from build123d import *

# Parameters (mm, degrees)
SKETCH1_W           = 30
SKETCH1_H           = 36
BOSS_EXTRUDE1_DEPTH = 30
SKETCH3_R           = 12.375
CUT_EXTRUDE1_DEPTH  = 40
SKETCH5_R           = 1.875
CUT_EXTRUDE2_DEPTH  = 40
CUT_EXTRUDE3_START  = 15
SKETCH7_W           = 36
SKETCH7_H           = 15
CUT_EXTRUDE3_DEPTH  = 31
SKETCH8_W           = 9.5
SKETCH8_H           = 22
CUT_EXTRUDE4_DEPTH  = 10


with BuildPart() as part:
    # Sketch1 → Boss-Extrude1 (new body)
    with BuildSketch(Plane(origin=(0, 0, 0), x_dir=(1, 0, 0), z_dir=(0, 1, 0))):
        Rectangle(SKETCH1_W, SKETCH1_H)
    extrude(amount=BOSS_EXTRUDE1_DEPTH)

    # Sketch3 → Cut-Extrude1 (cut)
    with BuildSketch(Plane(origin=(15, 0, 0), x_dir=(0, 0, -1), z_dir=(1, 0, 0))):
        with Locations((0, 15)):
            Circle(SKETCH3_R)
    extrude(amount=-CUT_EXTRUDE1_DEPTH, mode=Mode.SUBTRACT)

    # Sketch5 → Cut-Extrude2 (cut)
    with BuildSketch(Plane(origin=(0, 30, 0), x_dir=(1, 0, 0), z_dir=(0, 1, 0))):
        with Locations((-12.25, 15.25)):
            Circle(SKETCH5_R)
        with Locations((-12.25, -15.25)):
            Circle(SKETCH5_R)
        with Locations((12.25, -15.25)):
            Circle(SKETCH5_R)
        with Locations((12.25, 15.25)):
            Circle(SKETCH5_R)
    extrude(amount=-CUT_EXTRUDE2_DEPTH, mode=Mode.SUBTRACT)

    # Sketch7 → Cut-Extrude3 (cut, through all)
    with BuildSketch(Plane(origin=(0, 0, 0), x_dir=(0, 0, -1), z_dir=(1, 0, 0)).offset(CUT_EXTRUDE3_START)):
        with Locations((0, 7.5)):
            Rectangle(SKETCH7_W, SKETCH7_H)
    extrude(amount=-CUT_EXTRUDE3_DEPTH, mode=Mode.SUBTRACT)

    # Sketch8 → Cut-Extrude4 (cut)
    with BuildSketch(Plane(origin=(0, 30, 0), x_dir=(1, 0, 0), z_dir=(0, 1, 0))):
        with Locations((10.25, 0)):
            Rectangle(SKETCH8_W, SKETCH8_H)
    extrude(amount=-CUT_EXTRUDE4_DEPTH, mode=Mode.SUBTRACT)


solid = part.part
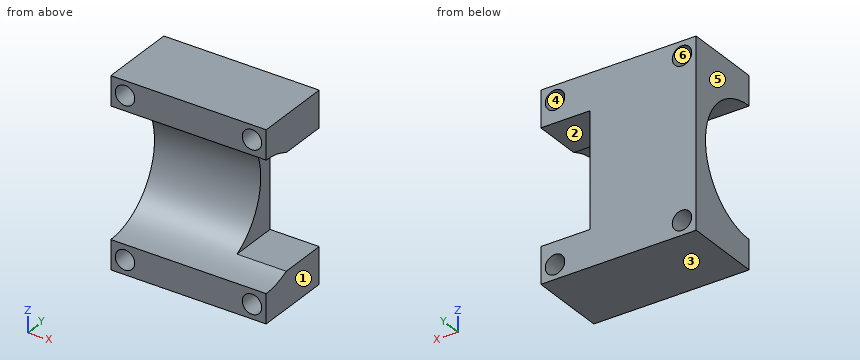
CAD build for the part. Positions are in the model's coordinates, mm. Face numbers are marked on the shaded views. A direction names the side the tool comes from. Round coordinates to 2 decimals unless told otherwise and drop trailing zeros. Order: outer loops, then holes, each group sorted by start corner. A loop starts at its lowest first (then second) coordinate and runs counter-clockwise, first axis right, second up. Notation, with made-up numbers: (-36.75, 24.5) -> (-10.75, 24.5) arc R28 ccw to (-10.75, 54.5) -> close; hole circle Ø1 at (-21.75, 2). An arc over 180 degrees is marked (long way). Write item = value, one per line. Start each with the question number.
(1) Pin check, flat tip, straight feed: P1, Ø8, axis at y = 20.5, z = -2, coming from the -X side. Stop position of the tip, or through.
(2) Pull direction Z, two halves, no side cores. Call the marked faces 3, 4, 5 and 6: released by +Z, released by -Z, zero draft, split by the parting line, or undercut.
(3) Cut at D-D, the plane y = 19. List the corners of the cut face in (x, z) (3 decimals).
(4) Which spindle directions (+Z, -Z, +X, -X, +Y, -Y) get a long thin tool onto all of the face, cutting with end or side? Do the marked faces 1 and 2. Say none if no direction does.
(5) Cut at C-C, the plane x = 12.25. List the corners of the cut face in (y, z) (3 decimals), then the cut area to 3 significant figures.
(6) Cut at B-B, the plane y = 28.25. List the corners of the cut face in (x, z) (3 decimals).
(7) Cut at A-A, the plane x = -12.25. List the corners of the cut face in (y, z) (3 decimals).
(8) Probe line 1 (X direction, y = 22.25, z = 15.25) (3 decimals); line 2 (Z direction, x = 12.25, y = 26.25) (3 decimals); line 3 (Z direction, x = -11.25, y = 28). List the from-to ranges inside material, lowest first. Write a range as [from, to].
Model answer:
q1.P1 = through
q2.face_3 = released by -Z
q2.face_4 = undercut
q2.face_5 = zero draft
q2.face_6 = undercut
q3.outline = (-15, -18) -> (15, -18) -> (15, -11.711) -> (-15, -11.711) -> close; (-15, 11.711) -> (15, 11.711) -> (15, 18) -> (-15, 18) -> close; hole circle Ø3.75 at (-12.25, -15.25); hole circle Ø3.75 at (-12.25, 15.25); hole circle Ø3.75 at (12.25, -15.25); hole circle Ø3.75 at (12.25, 15.25)
q4.face_1 = +Z, -Z, +X, +Y, -Y
q4.face_2 = +X, +Y, -Y
q5.outline = (15, -18) -> (30, -18) -> (30, -17.125) -> (15, -17.125) -> close; (15, -13.375) -> (30, -13.375) -> (30, -11) -> (20.669, -11) arc R12.375 cw to (15, -12.375) -> close; (15, 12.375) arc R12.375 cw to (20.669, 11) -> (30, 11) -> (30, 13.375) -> (15, 13.375) -> close; (15, 17.125) -> (30, 17.125) -> (30, 18) -> (15, 18) -> close
q5.area = 87.0 mm2
q6.outline = (-15, -18) -> (15, -18) -> (15, -11) -> (5.5, -11) -> (5.5, 11) -> (15, 11) -> (15, 18) -> (-15, 18) -> close; hole circle Ø3.75 at (-12.25, -15.25); hole circle Ø3.75 at (-12.25, 15.25); hole circle Ø3.75 at (12.25, -15.25); hole circle Ø3.75 at (12.25, 15.25)
q7.outline = (15, -18) -> (30, -18) -> (30, -17.125) -> (15, -17.125) -> close; (15, -13.375) -> (30, -13.375) -> (30, 13.375) -> (15, 13.375) -> (15, 12.375) arc R12.375 cw to (15, -12.375) -> close; (15, 17.125) -> (30, 17.125) -> (30, 18) -> (15, 18) -> close
q8.line_1 = [-15, -14.125], [-10.375, 10.375], [14.125, 15]
q8.line_2 = [-18, -17.125], [-13.375, -11], [11, 13.375], [17.125, 18]
q8.line_3 = [-18, -16.84], [-13.66, 13.66], [16.84, 18]
